Drawing for the job (mm, zero at the part's lowest x, y, z). A direction names the side the tool comes from. Round coordinates to 2 decimals unless told otherwise and drop trailing zeros. Write each loop counter-clockwise with the first axis right and the second up, starting at its lowest first coordinate (ties: lowest second). Pieces come first, ordered by that corner, then holes.
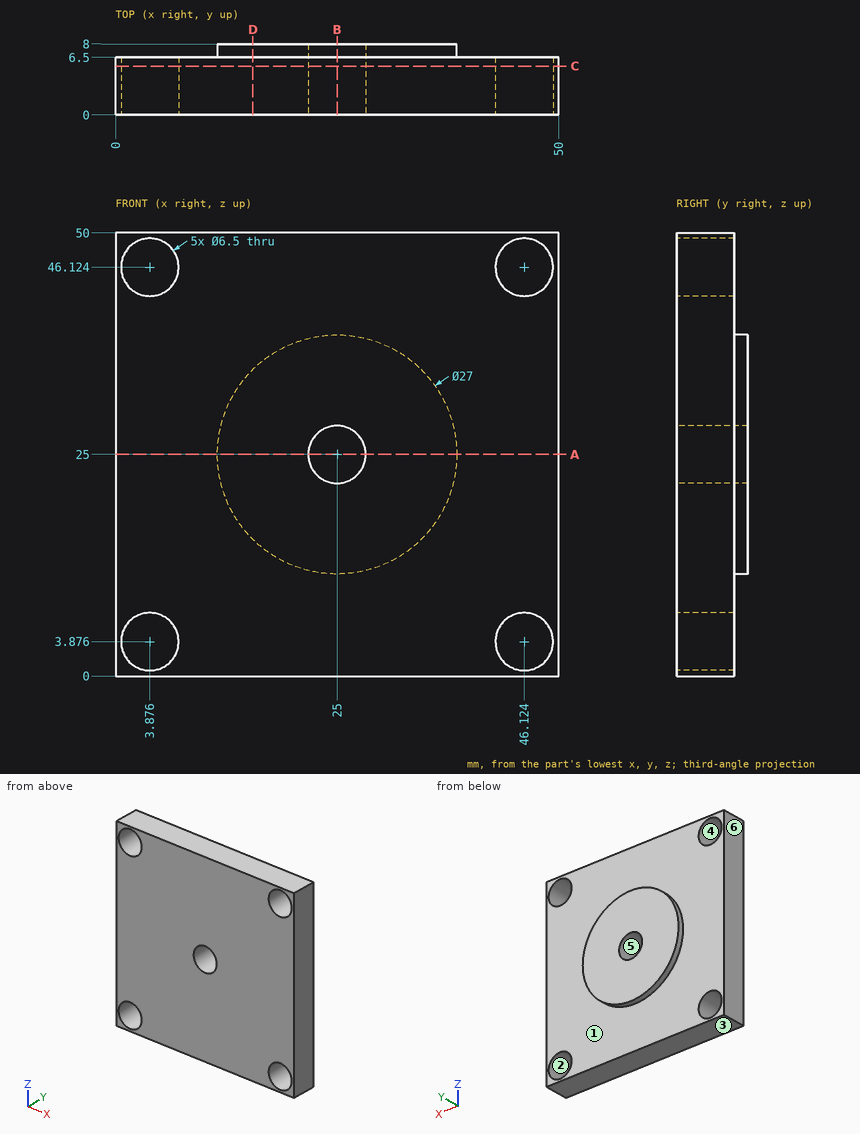
1) Which spindle directions (+Z, -Z, +X, -X, +Y, -Y) get a long thin tool onto all of the face, cutting with end or side? Do the marked faces 1 and 2. Say none if no direction does.
2) Wall check: probe 1 along Z at (x, y) = (46, 4); probe 2 along Z at (x, y) = (5, 0.5); probe 3 along X at (y, z) = (0.75, 3). Give the ranges that are in metal, low to high.
3) Cut at D-D on x = 15.5. List the corners of the cut face in (y, z).
4) Cut at C-C on y = 5.5. List the corners of the cut face in (x, z), and give its area (3 significant figures).
5) Cut at B-B on x = 25. List the corners of the cut face in (y, z), and give its area (4 significant figures).
6) Pull direction Z, two halves, no side cores. Call the marked faces 3, 4, 5 and 6: released by +Z, released by -Z, zero draft, split by the parting line, or undercut.
7) Cut at A-A on z = 25. List the corners of the cut face in (x, y), and give its area (4 significant figures).
8) Flat gauge pin, fed straight in: pin 1 Ø8.5 at (x, z) = (46.124, 3.876) entering from +Y. Where does the tip first touch, or does it go through?
Result sheet:
1. face 1: +Y
1. face 2: +Y, -Y
2. probe 1: z = 0 to 0.63, 7.12 to 42.88, 49.37 to 50
2. probe 2: z = 0 to 0.83, 6.93 to 43.07, 49.17 to 50
2. probe 3: x = 0 to 0.75, 7.01 to 42.99, 49.25 to 50
3. outline: (0, 0) - (6.5, 0) - (6.5, 15.41) - (8, 15.41) - (8, 34.59) - (6.5, 34.59) - (6.5, 50) - (0, 50) - close
4. outline: (0, 0) - (50, 0) - (50, 50) - (0, 50) - close; hole circle Ø6.5 at (3.88, 3.88); hole circle Ø6.5 at (3.88, 46.12); hole circle Ø6.5 at (25, 25); hole circle Ø6.5 at (46.12, 3.88); hole circle Ø6.5 at (46.12, 46.12)
4. area: 2,330 mm2
5. outline: (0, 0) - (6.5, 0) - (6.5, 11.5) - (8, 11.5) - (8, 21.75) - (0, 21.75) - close; (0, 28.25) - (8, 28.25) - (8, 38.5) - (6.5, 38.5) - (6.5, 50) - (0, 50) - close
5. area: 313.5 mm2
6. face 3: released by -Z
6. face 4: undercut
6. face 5: undercut
6. face 6: zero draft
7. outline: (0, 0) - (21.75, 0) - (21.75, 8) - (11.5, 8) - (11.5, 6.5) - (0, 6.5) - close; (28.25, 0) - (50, 0) - (50, 6.5) - (38.5, 6.5) - (38.5, 8) - (28.25, 8) - close
7. area: 313.5 mm2
8. pin 1: stops at y = 6.5
